Could you check a few things on this model? Use its own coordinates, in mm. Give positions to 0.01 mm unless a question says otherwise; leave off trailing zeros. Loops run counter-clockwise (first coordinate to the right, second up) from the corner with the lowest first, then second, coordinate; pieces in that order, holes last. Notation, with made-up numbers: (-15, 11.25) -> (-9, 11.25) arc R20 cw to (-9, 46.25) -> close; hole circle Ø9 at (-22, 84.25). An arc over 180 degrees is marked (long way). Write each question's results on one line, items separated by ' | '. Start each with the question number.
Q1. Will these pins go through, and if not, where does the flat tip stop? P1, Ø4.5, axis at x = -15.15, y = -32.11, coming from the -Z side; P2, Ø4, axis at y = -22, z = 8.5, coming from the -X side; P3, Ø1, axis at x = -10, z = 6, coming from the -Y side; P4, Ø2, axis at x = -20, z = 4.5, coming from the -Y side.
Q2. If we section it at D-D, the plane z = 6.75: List the corners of the cut face in (x, y) for me, plus the area to 3 significant figures.
Q3. If we section it at C-C, the plane y = -9.5: List the corners of the cut face in (x, z) for me, plus the area to 3 significant figures.
Q4. If I drill on line 1 along X through (y, z) = (-34, 9.75); line 2 along Y through (x, z) = (-22.5, 7.25); line 3 along X through (y, z) = (-19, 3), over which ranges is the centre line in solid material (lowest first)?
Q5. We'd pull the mould along X, two halves only. Please class faces 1 (the face through (-46.535, -16.708, 4.93)), 2 (the face through (-27.54, -33.07, 4.93)), 3 (the face through (-22, -17, 0)): released by +X, released by -X, zero draft, split by the parting line, or undercut.
Q6. If we section it at B-B, the plane y = -20: List the corners of the cut face in (x, z) for me, plus the area to 3 significant figures.
Q7. If we section it at A-A, the plane x = -22.5: List the corners of the cut face in (y, z) for me.
from build123d import *

# Parameters (mm, degrees)
CROQUIS1_R              = 2.5
SALIENTE_EXTRUIR1_DEPTH = 10


with BuildPart() as part:
    # Croquis1 → Saliente-Extruir1 (new body)
    with BuildSketch(Plane.XY):
        with BuildLine():
            Line((-45, 8), (0, 8))
            ThreePointArc((0, 8), (6.679829127, 4.402258834), (7.351584195, -3.15502929))
            Line((7.351584195, -3.15502929), (-4.121039512, -29.887573226))
            ThreePointArc((-4.121039512, -29.887573226), (-22.5, -42), (-40.878960488, -29.887573226))
            Line((-40.878960488, -29.887573226), (-52.351584195, -3.15502929))
            ThreePointArc((-52.351584195, -3.15502929), (-51.679829127, 4.402258834), (-45, 8))
        make_face()
        with Locations((-22.5, -9.5)):
            Circle(CROQUIS1_R, mode=Mode.SUBTRACT)
        with Locations((-10.611793546, -18.13728757)):
            Circle(CROQUIS1_R, mode=Mode.SUBTRACT)
        with Locations((-15.152684346, -32.11271243)):
            Circle(CROQUIS1_R, mode=Mode.SUBTRACT)
        with Locations((-29.847315654, -32.11271243)):
            Circle(CROQUIS1_R, mode=Mode.SUBTRACT)
        with Locations((-34.388206454, -18.13728757)):
            Circle(CROQUIS1_R, mode=Mode.SUBTRACT)
    extrude(amount=SALIENTE_EXTRUIR1_DEPTH)


solid = part.part
Final values:
1) P1: passes through | P2: stops at x = -45.12 | P3: stops at y = -38 | P4: stops at y = -41.94
2) outline: (-52.35, -3.16) -> (-40.88, -29.89) arc R20 ccw to (-4.12, -29.89) -> (7.35, -3.16) arc R8 ccw to (0, 8) -> (-45, 8) arc R8 ccw to start; hole circle Ø5 at (-34.39, -18.14); hole circle Ø5 at (-29.85, -32.11); hole circle Ø5 at (-22.5, -9.5); hole circle Ø5 at (-15.15, -32.11); hole circle Ø5 at (-10.61, -18.14) | area: 2,160 mm²
3) outline: (-49.63, 0) -> (-25, 0) -> (-25, 10) -> (-49.63, 10) -> close; (-20, 0) -> (4.63, 0) -> (4.63, 10) -> (-20, 10) -> close | area: 493 mm²
4) line 1: x = -38.5 to -31.49, -28.21 to -16.79, -13.51 to -6.5 | line 2: y = -42 to -12, -7 to 8 | line 3: x = -45.55 to -36.73, -32.04 to -12.96, -8.27 to 0.55
5) face 1: released by -X | face 2: undercut | face 3: zero draft
6) outline: (-45.12, 0) -> (-36.06, 0) -> (-36.06, 10) -> (-45.12, 10) -> close; (-32.72, 0) -> (-12.28, 0) -> (-12.28, 10) -> (-32.72, 10) -> close; (-8.94, 0) -> (0.12, 0) -> (0.12, 10) -> (-8.94, 10) -> close | area: 386 mm²
7) outline: (-42, 0) -> (-12, 0) -> (-12, 10) -> (-42, 10) -> close; (-7, 0) -> (8, 0) -> (8, 10) -> (-7, 10) -> close
